Here's how the part is built. I have some questions about the finished solid (model axes, mm). Face numbers are marked on the shaded views. Give positions to 0.01 mm unless a question says otherwise; leave off trailing zeros. Write each loop counter-clockwise with the first axis right and the second up, starting at its lowest first coordinate (ties: lowest second). Pieces come first, ordered by that corner, then holes. Notation, with made-up numbers: (72, 17.25) -> (106, 17.25) arc R17 ccw to (106, 37.25) -> close; hole circle Ø2 at (19.25, 50). An arc over 180 degrees is marked (long way). Put each result on its own line as item: value. Start each with the question number.
from build123d import *

# Parameters (mm, degrees)
F0_W          = 2000
F0_H          = 1796
F1_DEPTH      = 40
F2_W          = 2000
F2_H          = 680
F3_DEPTH      = 850
F4_W          = 1920
F4_H          = 640
F5_DEPTH      = 40.001
F5_DEPTH_BACK = 850.001
F7_DEPTH      = 2000.001
F8_W          = 1920
F8_H          = 400
F8_H_2        = 370
F9_DEPTH      = 680.001
F11_DEPTH     = 40
F12_W         = 40
F12_H         = 1076
F13_DEPTH     = 40
F14_W         = 400
F14_H         = 40
F15_DEPTH     = 3
F17_DEPTH     = 2
F19_DEPTH     = 2


with BuildPart() as f1:
    # F0 (on Front) → F1 (new body)
    with BuildSketch(Plane.XZ):
        Rectangle(F0_W, F0_H)
    extrude(amount=F1_DEPTH)

    # F2 (on face) → F3 (join)
    with BuildSketch(Plane(origin=(0, 0, 0), x_dir=(-1, 0, 0), z_dir=(0, 1, 0))):
        with Locations((0, -558)):
            Rectangle(F2_W, F2_H)
    extrude(amount=F3_DEPTH)

    # F4 (on face) → F5 (cut, two sides)
    with BuildSketch(Plane(origin=(0, 0, 0), x_dir=(-1, 0, 0), z_dir=(0, 1, 0))) as f5_sk:
        with Locations((0, -578)):
            Rectangle(F4_W, F4_H)
        Polygon((-161.4213562373, -218), (-20, -76.5786437627), (-20, 716.5786437627), (-161.4213562373, 858), (-818.5786437627, 858), (-960, 716.5786437627), (-960, -76.5786437627), (-818.5786437627, -218), align=None)
        Polygon((20, 716.5786437627), (20, -76.5786437627), (161.4213562373, -218), (818.5786437627, -218), (960, -76.5786437627), (960, 716.5786437627), (818.5786437627, 858), (161.4213562373, 858), align=None)
    extrude(amount=-F5_DEPTH, mode=Mode.SUBTRACT)
    extrude(f5_sk.sketch, amount=F5_DEPTH_BACK, mode=Mode.SUBTRACT)

    # F6 (on face) → F7 (cut, through all)
    with BuildSketch(Plane(origin=(-1000, 0, 0), x_dir=(0, -1, 0), z_dir=(-1, 0, 0))):
        Polygon((-63.8319580969, -858), (-810, -258), (-810, -858), align=None)
        Polygon((0, -858), (0, -258), (-746.1680419031, -258), align=None)
    extrude(amount=-F7_DEPTH, mode=Mode.SUBTRACT)

    # F8 (on face) → F9 (cut, through all)
    with BuildSketch(Plane.XY.offset(-218)):
        with Locations((0, 650)):
            Rectangle(F8_W, F8_H)
        with Locations((0, 225)):
            Rectangle(F8_W, F8_H_2)
    extrude(amount=-F9_DEPTH, mode=Mode.SUBTRACT)

    # F10 (on face) → F11 (join)
    with BuildSketch(Plane.XZ.offset(40)):
        Polygon((72.1110255093, -258), (0, -258), (960, -898), (960, -849.9259829938), align=None)
        Polygon((-960, -898), (0, -258), (-72.1110255093, -258), (-960, -849.9259829938), align=None)
    extrude(amount=-F11_DEPTH)

    # F12 (on face) → F13 (join)
    with BuildSketch(Plane.XZ.offset(40)):
        with Locations((-710, 320)):
            Rectangle(F12_W, F12_H)
        with Locations((-270, 320)):
            Rectangle(F12_W, F12_H)
        with Locations((270, 320)):
            Rectangle(F12_W, F12_H)
        with Locations((710, 320)):
            Rectangle(F12_W, F12_H)
    extrude(amount=-F13_DEPTH)

    # F14 (on face) → F15 (join)
    with BuildSketch(Plane(origin=(0, 0, 0), x_dir=(-1, 0, 0), z_dir=(0, 1, 0))):
        with Locations((490, 745)):
            Rectangle(F14_W, F14_H)
        with BuildLine():
            Line((327, 748.5), (337, 748.5))
            Line((337, 748.5), (347, 748.5))
            ThreePointArc((347, 748.5), (350.5, 745), (347, 741.5))
            Line((347, 741.5), (337, 741.5))
            Line((337, 741.5), (327, 741.5))
            ThreePointArc((327, 741.5), (323.5, 745), (327, 748.5))
        make_face(mode=Mode.SUBTRACT)
        with BuildLine():
            Line((627, 748.5), (637, 748.5))
            Line((637, 748.5), (647, 748.5))
            ThreePointArc((647, 748.5), (650.5, 745), (647, 741.5))
            Line((647, 741.5), (637, 741.5))
            Line((637, 741.5), (627, 741.5))
            ThreePointArc((627, 741.5), (623.5, 745), (627, 748.5))
        make_face(mode=Mode.SUBTRACT)
        with Locations((490, 445)):
            Rectangle(F14_W, F14_H)
        with BuildLine():
            Line((327, 448.5), (337, 448.5))
            Line((337, 448.5), (347, 448.5))
            ThreePointArc((347, 448.5), (350.5, 445), (347, 441.5))
            Line((347, 441.5), (337, 441.5))
            Line((337, 441.5), (327, 441.5))
            ThreePointArc((327, 441.5), (323.5, 445), (327, 448.5))
        make_face(mode=Mode.SUBTRACT)
        with BuildLine():
            Line((627, 448.5), (637, 448.5))
            Line((637, 448.5), (647, 448.5))
            ThreePointArc((647, 448.5), (650.5, 445), (647, 441.5))
            Line((647, 441.5), (637, 441.5))
            Line((637, 441.5), (627, 441.5))
            ThreePointArc((627, 441.5), (623.5, 445), (627, 448.5))
        make_face(mode=Mode.SUBTRACT)
        with Locations((-490, 745)):
            Rectangle(F14_W, F14_H)
        with BuildLine():
            Line((-647, 748.5), (-637, 748.5))
            Line((-637, 748.5), (-627, 748.5))
            ThreePointArc((-627, 748.5), (-623.5, 745), (-627, 741.5))
            Line((-627, 741.5), (-637, 741.5))
            Line((-637, 741.5), (-647, 741.5))
            ThreePointArc((-647, 741.5), (-650.5, 745), (-647, 748.5))
        make_face(mode=Mode.SUBTRACT)
        with BuildLine():
            Line((-347, 748.5), (-337, 748.5))
            Line((-337, 748.5), (-327, 748.5))
            ThreePointArc((-327, 748.5), (-323.5, 745), (-327, 741.5))
            Line((-327, 741.5), (-337, 741.5))
            Line((-337, 741.5), (-347, 741.5))
            ThreePointArc((-347, 741.5), (-350.5, 745), (-347, 748.5))
        make_face(mode=Mode.SUBTRACT)
        with Locations((-490, 445)):
            Rectangle(F14_W, F14_H)
        with BuildLine():
            Line((-647, 448.5), (-637, 448.5))
            Line((-637, 448.5), (-627, 448.5))
            ThreePointArc((-627, 448.5), (-623.5, 445), (-627, 441.5))
            Line((-627, 441.5), (-637, 441.5))
            Line((-637, 441.5), (-647, 441.5))
            ThreePointArc((-647, 441.5), (-650.5, 445), (-647, 448.5))
        make_face(mode=Mode.SUBTRACT)
        with BuildLine():
            Line((-347, 448.5), (-337, 448.5))
            Line((-337, 448.5), (-327, 448.5))
            ThreePointArc((-327, 448.5), (-323.5, 445), (-327, 441.5))
            Line((-327, 441.5), (-337, 441.5))
            Line((-337, 441.5), (-347, 441.5))
            ThreePointArc((-347, 441.5), (-350.5, 445), (-347, 448.5))
        make_face(mode=Mode.SUBTRACT)
    extrude(amount=-F15_DEPTH)

    # F16 (on face) → F17 (join)
    with BuildSketch(Plane(origin=(-1000, 0, 0), x_dir=(0, -1, 0), z_dir=(-1, 0, 0))):
        Polygon((40, 392), (-263.0999778007, -258), (40, -258), align=None)
    extrude(amount=-F17_DEPTH)

    # F18 (on face) → F19 (join)
    with BuildSketch(Plane.YZ.offset(1000)):
        Polygon((-40, -258), (263.0999778007, -258), (-40, 392), align=None)
    extrude(amount=-F19_DEPTH)


solid = f1.part
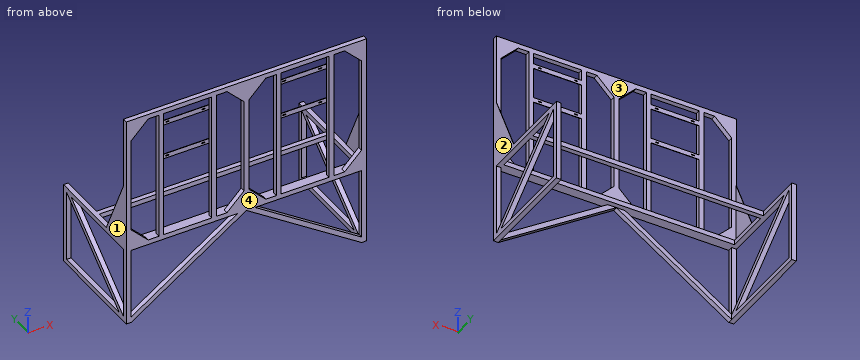
1) I want a section at A-A, the plane z = 685.5. Write out the boundary of the cut face in (x, y).
2) I'm going to push flat-ended pins straight in: pin 1 Ø2.5 at (x, y) = (531, -2) entering from -Z; pin 2 Ø0.9 at (x, y) = (640, -2) entering from -Z; pin 3 Ø12 at (x, y) = (-435, -25) entering from -Z. Where does each tip first touch, or does it pass through?
3) I want a section at D-D, the plane z = -739. State how many separate pieces and enclosed holes the cut face has, and give its area (3 significant figures).
4) I want a section at B-B, the plane y = 192.5. Write out the boundary of the cut face in (x, z), and give its area (3 significant figures).
5) I want a section at C-C, the plane x = 440.5. Write out the boundary of the cut face in (y, z), and give its area (3 significant figures).
6) Thinking about a two-plate mould opening in X: for the marked faces 1, 2, 3 and 4, which applies, released by +X, released by -X, zero draft, split by the parting line, or undercut?
7) I need wall thicknesses on probe 1 along X at (y, z) = (358, -219); probe 2 along Y at (x, z) = (346, -256.5); probe 3 along X at (y, z) = (88.5, 66.5). Which ranges of each line are inside material? Lowest first, please.
Established:
1. outline: (-1000, -40) -> (-960, -40) -> (-960, 0) -> (-1000, 0) -> close; (-730, -40) -> (-690, -40) -> (-690, 0) -> (-730, 0) -> close; (-290, -40) -> (-250, -40) -> (-250, 0) -> (-290, 0) -> close; (-20, -40) -> (20, -40) -> (20, 0) -> (-20, 0) -> close; (250, -40) -> (290, -40) -> (290, 0) -> (250, 0) -> close; (690, -40) -> (730, -40) -> (730, 0) -> (690, 0) -> close; (960, -40) -> (1000, -40) -> (1000, 0) -> (960, 0) -> close
2. pin 1: stops at z = -612.83
2. pin 2: stops at z = -684.97
2. pin 3: stops at z = -552
3. separate pieces: 8
3. enclosed holes: 0
3. area: 17,300 mm2
4. outline: (-1000, -898) -> (-960, -898) -> (-960, -858) -> (-1000, -858) -> close; (-1000, -754.54) -> (-960, -754.54) -> (-960, -703.21) -> (-1000, -703.21) -> close; (-1000, -258) -> (-960, -258) -> (-960, -218) -> (-998, -218) -> (-998, -106.6) -> (-1000, -106.6) -> close; (960, -898) -> (1000, -898) -> (1000, -858) -> (960, -858) -> close; (960, -754.54) -> (1000, -754.54) -> (1000, -703.21) -> (960, -703.21) -> close; (960, -258) -> (1000, -258) -> (1000, -106.6) -> (998, -106.6) -> (998, -218) -> (960, -218) -> close
4. area: 11,000 mm2
5. outline: (-40, -551.67) -> (0, -551.67) -> (0, -503.59) -> (-40, -503.59) -> close; (-40, -258) -> (40, -258) -> (40, -218) -> (-40, -218) -> close; (-40, 858) -> (0, 858) -> (0, 898) -> (-40, 898) -> close; (-3, 425) -> (0, 425) -> (0, 465) -> (-3, 465) -> close; (-3, 725) -> (0, 725) -> (0, 765) -> (-3, 765) -> close; (410, -258) -> (450, -258) -> (450, -218) -> (410, -218) -> close
5. area: 8,560 mm2
6. face 1: released by -X
6. face 2: released by +X
6. face 3: undercut
6. face 4: zero draft
7. probe 1: x = -1000 to -960, 960 to 1000
7. probe 2: y = -40 to 40, 410 to 450
7. probe 3: x = -1000 to -998, 998 to 1000
